Source: CAD feature listing. Evaluate the final solid. Frame: model axes, mm. A direction names the side the tool comes from. Give positions to 0.01 mm unless a question says otherwise; leave off trailing zeros. Loops run counter-clockwise (first coordinate to the right, second up) from the corner with the lowest first, then second, coordinate; pieces in that order, holes last. Notation, with made-up numbers: M -7,55.25 L 51,55.25 A8 cw 51,66.25 Z; hole C 42,10 d3. An arc over 180 degrees is marked long. Write item = value, one per line.
from build123d import *

# Parameters (mm, degrees)
ESQUISSE1_R                  = 5.75
ESQUISSE1_R_2                = 1.6
BOSS_EXTRU_1_DEPTH           = 5
ESQUISSE2_R                  = 3
ENL_V_MAT_EXTRU_1_DEPTH      = 3
ENL_V_START                  = -3
ESQUISSE3_R                  = 5.75
ESQUISSE3_R_2                = 4.5
ENL_V_MAT_EXTRU_2_DEPTH      = 3
BOSS_EXTRU_2_DEPTH           = 2
R_P_TITION_CIRCULAIRE1_COUNT = 4
ESQUISSE5_R                  = 0.75
ENL_V_MAT_EXTRU_3_DEPTH      = 3
R_P_TITION_CIRCULAIRE2_COUNT = 4
BOSS_EXTRU_3_DEPTH           = 3
R_P_TITION_CIRCULAIRE3_COUNT = 28
ENL_V_START_2                = -1
ESQUISSE7_R                  = 3
ESQUISSE7_R_2                = 1.6
ENL_V_MAT_EXTRU_4_DEPTH      = 1
ESQUISSE8_R                  = 4.7
ESQUISSE8_R_2                = 3.4
ENL_V_MAT_EXTRU_5_DEPTH      = 1


with BuildPart() as part:
    # Esquisse1 → Boss.-Extru.1 (new body)
    with BuildSketch(Plane.XY):
        Circle(ESQUISSE1_R)
        Circle(ESQUISSE1_R_2, mode=Mode.SUBTRACT)
    extrude(amount=BOSS_EXTRU_1_DEPTH)

    # Esquisse2 → Enlèv. mat.-Extru.1 (cut)
    with BuildSketch(Plane.XY.offset(5)):
        Circle(ESQUISSE2_R)
    extrude(amount=-ENL_V_MAT_EXTRU_1_DEPTH, mode=Mode.SUBTRACT)

    # Esquisse3 → Enlèv. mat.-Extru.2 (cut)
    with BuildSketch(Plane.XY.offset(5).offset(ENL_V_START)):
        Circle(ESQUISSE3_R)
        Circle(ESQUISSE3_R_2, mode=Mode.SUBTRACT)
    extrude(amount=ENL_V_MAT_EXTRU_2_DEPTH, mode=Mode.SUBTRACT)

    # Esquisse4 → Boss.-Extru.2 (add)
    with BuildSketch(Plane(origin=(0, 0, 0), x_dir=(-1, 0, 0), z_dir=(0, 0, -1))):
        with BuildLine():
            Line((-4.3, 3.817394399), (-2.475852955, 16.846629695))
            ThreePointArc((-2.475852955, 16.846629695), (0, 19), (2.475852955, 16.846629695))
            Line((2.475852955, 16.846629695), (4.3, 3.817394399))
            ThreePointArc((4.3, 3.817394399), (0, 5.75), (-4.3, 3.817394399))
        make_face()
    boss_extru_2 = extrude(amount=-BOSS_EXTRU_2_DEPTH)

    # Répétition circulaire1: Boss.-Extru.2 ×4 about axis
    r_p_tition_circulaire1_axis = Axis((0, 0, 0), (0, 0, 1))
    for i in range(1, R_P_TITION_CIRCULAIRE1_COUNT):
        add(boss_extru_2.rotate(r_p_tition_circulaire1_axis, i * 360 / R_P_TITION_CIRCULAIRE1_COUNT))

    # Esquisse5 → Enlèv. mat.-Extru.3 (cut)
    with BuildSketch(Plane(origin=(0, 0, 0), x_dir=(-1, 0, 0), z_dir=(0, 0, -1))):
        with Locations((0, 7)):
            Circle(ESQUISSE5_R)
        with Locations((0, 10)):
            Circle(ESQUISSE5_R)
        with Locations((0, 13)):
            Circle(ESQUISSE5_R)
        with Locations((0, 16)):
            Circle(ESQUISSE5_R)
    enl_v_mat_extru_3 = extrude(amount=-ENL_V_MAT_EXTRU_3_DEPTH, mode=Mode.SUBTRACT)

    # Répétition circulaire2: Enlèv. mat.-Extru.3 ×4 about axis
    r_p_tition_circulaire2_axis = Axis((0, 0, 0), (0, 0, 1))
    for i in range(1, R_P_TITION_CIRCULAIRE2_COUNT):
        add(enl_v_mat_extru_3.rotate(r_p_tition_circulaire2_axis, i * 360 / R_P_TITION_CIRCULAIRE2_COUNT), mode=Mode.SUBTRACT)

    # Esquisse6 → Boss.-Extru.3 (add)
    with BuildSketch(Plane.XY.offset(5)):
        Polygon((-0.3, 3), (0, 2.7), (0.3, 3), align=None)
    boss_extru_3 = extrude(amount=-BOSS_EXTRU_3_DEPTH)

    # Répétition circulaire3: Boss.-Extru.3 ×28 about axis
    r_p_tition_circulaire3_axis = Axis((0, 0, 0), (0, 0, 1))
    for i in range(1, R_P_TITION_CIRCULAIRE3_COUNT):
        add(boss_extru_3.rotate(r_p_tition_circulaire3_axis, i * 360 / R_P_TITION_CIRCULAIRE3_COUNT))

    # Esquisse7 → Enlèv. mat.-Extru.4 (cut)
    with BuildSketch(Plane(origin=(0, 0, 0), x_dir=(-1, 0, 0), z_dir=(0, 0, -1)).offset(ENL_V_START_2)):
        Circle(ESQUISSE7_R)
        Circle(ESQUISSE7_R_2, mode=Mode.SUBTRACT)
    extrude(amount=ENL_V_MAT_EXTRU_4_DEPTH, mode=Mode.SUBTRACT)

    # Esquisse8 → Enlèv. mat.-Extru.5 (cut)
    with BuildSketch(Plane(origin=(0, 0, 0), x_dir=(-1, 0, 0), z_dir=(0, 0, -1))):
        Circle(ESQUISSE8_R)
        Circle(ESQUISSE8_R_2, mode=Mode.SUBTRACT)
    extrude(amount=-ENL_V_MAT_EXTRU_5_DEPTH, mode=Mode.SUBTRACT)


solid = part.part
1. First-contact query: pin 1 Ø1.2 at (x, y) = (0, -13) entering from +Z; pin 2 Ø8 at (x, y) = (-2.5, 15) entering from +Z; pin 3 Ø1.5 at (x, z) = (-1, 2) entering from +Y; pin 4 Ø2 at (x, z) = (4.5, 3.5) entering from +Y. Flat tips, straight axial feed; report the tip coordinate or a pass-through.
Derived:
pin_1 = through
pin_2 = 2
pin_3 = 18.99
pin_4 = 2.83
2. Cut plane C-C, the plane x = 14.5. Return the cut outline in (y, z), then the cut area to 3 significant figures.
Derived:
outline = M -2.8,0 L 2.8,0 L 2.8,2 L -2.8,2 Z
area = 11.2 mm²
3. Cut plane A-A, the plane x = -16. Return the cut outline in (y, z).
Derived:
outline = M -2.59,0 L -0.75,0 L -0.75,2 L -2.59,2 Z; M 0.75,0 L 2.59,0 L 2.59,2 L 0.75,2 Z
4. Material intervals for probe 1 along Z at (x, y) = (15, 1.5); probe 2 along X at (y, z) = (-10, 1.2); probe 3 along X at (y, z) = (-16, 1.1), sorted ascending. Write a range as from..to.
Derived:
probe_1 = 0..2
probe_2 = -3.43..-0.75, 0.75..3.43
probe_3 = -2.59..-0.75, 0.75..2.59
5. Cut plane D-D, the plane y = -5.5. Return the cut outline in (x, z), then the cut area to 3 significant figures.
Derived:
outline = M -4.06,0 L 4.06,0 L 4.06,2 L -4.06,2 Z
area = 16.3 mm²
6. Pull-direction query (Y, two-part tool) for faces 3 (the flat face through (10.46, -3.37, 0.99)), 4 (the cylindrical face through (-0.098, -13.744, 0.986)), 5 (the flat face through (3.37, 10.46, 0.99)); classes: +Y half, -Y half, draft (parallel to the pull), parting line (faces both ways), or undercut.
Derived:
face_3 = -Y half
face_4 = undercut
face_5 = +Y half
7. Reachability of faces 1 (the flat face through (1.3, -1.3, 2)), 2 (the cylindrical face through (6.268, -0.163, 0.986)) from +Z, -Z, +X, -X, +Y, -Y: full face, straight path, thin tool, end or side. Return the list, or none.
Derived:
face_1 = +Z
face_2 = +Z, -Z
